Part print with two shaded views. Sizes in mm from the minimum x, y, z corner. A direction names the side the tool comes from. Round coordinates to 2 decimals unless told otherwise and drop trailing zeros. Write each loop counter-clockwise with the first axis right and the second up, starting at its lowest first coordinate (ties: lowest second). Pieces come first, ordered by that corner, then holes. Notation, with made-up numbers: (29.5, 42.5) -> (38.5, 42.5) arc R13 cw to (38.5, 47.5) -> close; hole circle Ø10 at (-27, 20.5). An arc over 180 degrees is marked (long way). Return JSON: item names as keys, results as strings. Group by question number.
(1) Tool access for the marked faces 1, 2 and 3: list every direction of +Z, -Z, +X, -X, +Y, -Y with a clear straight run to the whole face (end or side of a thin tool).
(2) Drop flat-ended pins along their axis: pin 1 Ø12 at (x, z) = (19, 74) entering from +Y; pin 2 Ø1 at (x, z) = (69.5, 4.5) entering from +Y; pin 3 Ø3 at (y, z) = (13, 85.5) entering from -X. Give the stop position or say it passes through.
(3) Drill centre lines: L1, parallel to X at y = 16, z = 38.5; L2, parallel to Z at x = 102, y = 2.25; L3, parallel to Y at x = 55, z = 53. Where is each one in solid material? Low to high. Write a range as from..to.
(4) Saw through at C-C (z = 70.5). List the corners of the cut face in (x, y).
(5) Saw through at B-B (y = 11.75). List the corners of the cut face in (x, z).
(6) Mould opens along X. For the marked faces 4, 5 and 6 say: +X half, -X half, draft (parallel to the pull), parting line (faces both ways), or undercut.
(7) Saw through at A-A (x = 71). List the corners of the cut face in (y, z), plus the area to 3 significant figures.
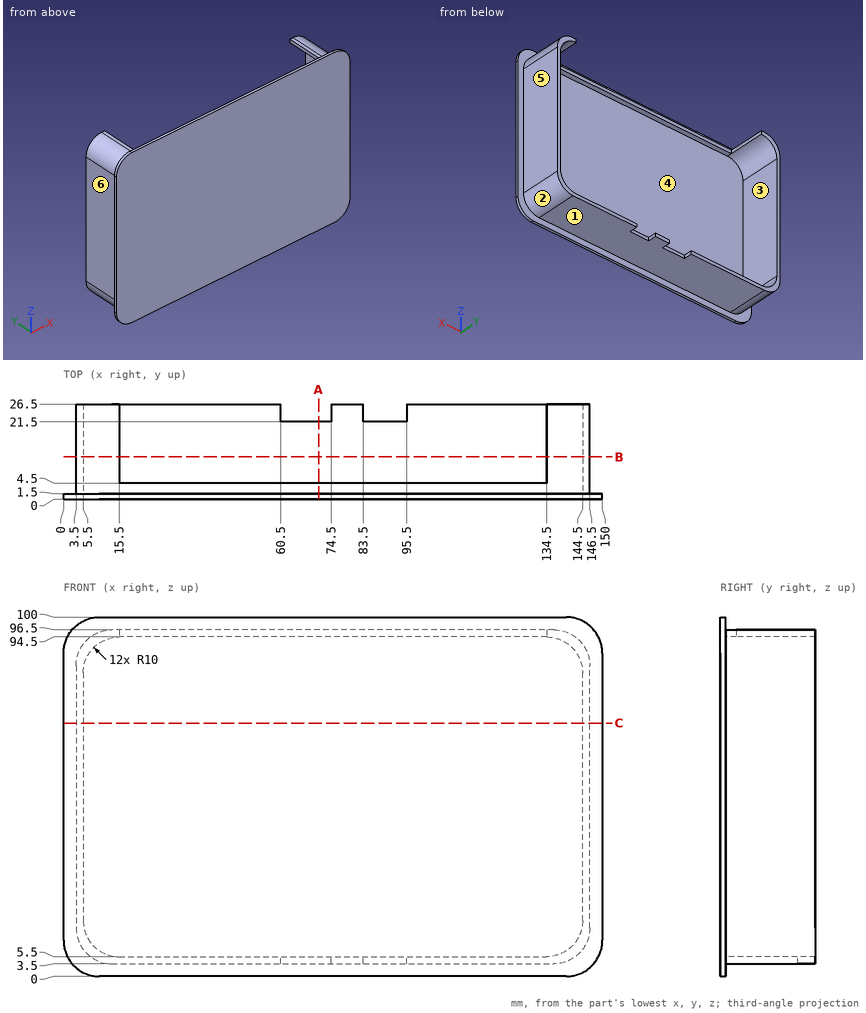
Computed values:
{
 "1": {"face 1": "-Z, +X, -X, +Y", "face 2": "-Z, +X, +Y", "face 3": "+Y"},
 "2": {"pin 1": "y = 1.5", "pin 2": "y = 21.5", "pin 3": "x = 3.5"},
 "3": {"L1": "3.5..5.5, 144.5..146.5", "L2": "3.5..5.5, 94.5..96.5", "L3": "0..1.5"},
 "4": {"outline": "(0, 0) -> (150, 0) -> (150, 1.5) -> (146.5, 1.5) -> (146.5, 26.5) -> (144.5, 26.5) -> (144.5, 1.5) -> (5.5, 1.5) -> (5.5, 26.5) -> (3.5, 26.5) -> (3.5, 1.5) -> (0, 1.5) -> close"},
 "5": {"outline": "(3.5, 13.5) arc R10 ccw to (13.5, 3.5) -> (136.5, 3.5) arc R10 ccw to (146.5, 13.5) -> (146.5, 86.5) arc R10 ccw to (136.5, 96.5) -> (134.5, 96.5) -> (134.5, 94.5) arc R10 cw to (144.5, 84.5) -> (144.5, 15.5) arc R10 cw to (134.5, 5.5) -> (15.5, 5.5) arc R10 cw to (5.5, 15.5) -> (5.5, 84.5) arc R10 cw to (15.5, 94.5) -> (15.5, 96.5) -> (13.5, 96.5) arc R10 ccw to (3.5, 86.5) -> close"},
 "6": {"face 4": "undercut", "face 5": "+X half", "face 6": "-X half"},
 "7": {"outline": "(0, 0) -> (1.5, 0) -> (1.5, 3.5) -> (21.5, 3.5) -> (21.5, 5.5) -> (1.5, 5.5) -> (1.5, 94.5) -> (4.5, 94.5) -> (4.5, 96.5) -> (1.5, 96.5) -> (1.5, 100) -> (0, 100) -> close", "area": "196 mm2"}
}
